The model under review builds one solid part; all positions refer to its coordinate system, in mm. Face numbers are marked on the shaded views. A direction names the side the tool comes from. Round coordinates to 2 decimals unless told otherwise and drop trailing zeros. Write each loop counter-clockwise with the first axis right and the second up, starting at its lowest first coordinate (ties: lowest second). Pieces come first, ordered by that corner, then holes. Notation, with made-up numbers: (24.5, 77) -> (80.5, 77) arc R15 ccw to (80.5, 95) -> close; hole circle Ø7 at (21.5, 84.25). An arc over 180 degrees is marked (long way). Answer in a Markdown table with one row per item. Add a question column.
```python
from build123d import *

# Parameters (mm, degrees)
F0_W     = 60.6719590724
F0_H     = 22.7290727198
F1_DEPTH = 44.45
F2_T     = -5.08
F4_DEPTH = 5.08
F6_DEPTH = 5.08
F7_R     = 2.6371182677
F8_DEPTH = 55.245


with BuildPart() as f1:
    # F0 (on Front) → F1 (new body)
    with BuildSketch(Plane.XZ):
        with Locations((-0.4582479596, -0.0916495919)):
            Rectangle(F0_W, F0_H)
    extrude(amount=F1_DEPTH)

    # F2
    f2_openings = [f1.faces().sort_by_distance(p)[0] for p in [
        (-0.458248, -22.225, 11.272887),
    ]]
    offset(amount=F2_T, openings=f2_openings)

    # F3 (on face) → F4 (join)
    with BuildSketch(Plane.YZ.offset(29.8777315766)):
        Polygon((-23.583047092, 26.9575025886), (-44.45, 11.272886768), (0, 11.272886768), align=None)
    extrude(amount=-F4_DEPTH)

    # F5 (on face) → F6 (join)
    with BuildSketch(Plane(origin=(-30.7942274958, 0, 0), x_dir=(0, -1, 0), z_dir=(-1, 0, 0))):
        Polygon((23.8014105707, 26.3420511037), (0, 11.272886768), (44.45, 11.272886768), align=None)
    extrude(amount=-F6_DEPTH)

    # F7 (on face) → F8 (join)
    with BuildSketch(Plane.YZ.offset(-25.7142274958)):
        with Locations((-23.0470523238, 16.2523370236)):
            Circle(F7_R)
    extrude(amount=F8_DEPTH)


solid = f1.part
```
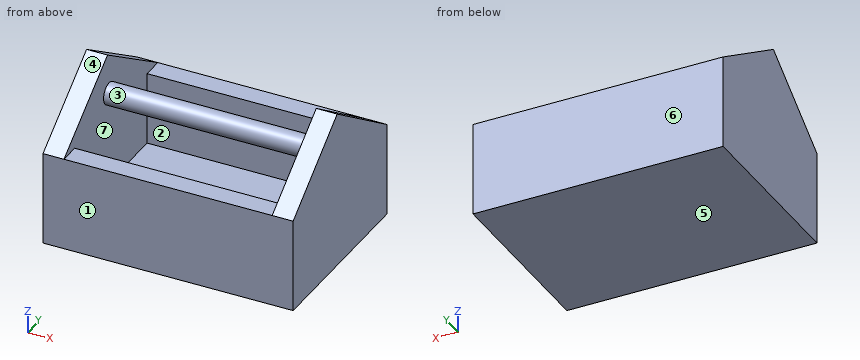
1. Mouldability with a two-part tool opening along Z and no side actions: class the marked faces 5, 6 and 7 as pulls with the +Z half, pulls with the -Z half, needs draft (parallel to the pull), parting line crosses it, or undercut.
2. Add section D-D on z = 12. Write out the cut boundary in (x, y).
3. Tool access review of the marked faces 1, 2, 3 and 4: name each direction out of +Z, -Z, +X, -X, +Y, -Y from which nothing blocks a thin tool from reaching the whole face with its end or side.
4. Add section B-B on y = -24.5. Write out the cut boundary in (x, z), plus the area to 3 significant figures.
5. Add section A-A on z = 4. Write out the cut boundary in (x, y).
6. Insertion check: pin 1 Ø4 at (x, y) = (-5, -41) entering from +Z; pin 2 Ø17 at (x, y) = (2.5, -26) entering from +Z. Each pin has a flat end and moves straight along its axis. Give the tip position at first contact, or say it passes through.
7. Add section C-C on x = -2. Write out the cut boundary in (y, z), plus the area to 3 significant figures.
8. For L1, parallel to X at y = -35.5, z = -3.5; L2, parallel to Y at x = -7, z = 9.5; L3, parallel to Z at x = 7.5, y = -37, list the stretches that pass through material, from the lowest coordinate up.
Filled in:
| question | item | result |
|---|---|---|
| 1 | face 5 | pulls with the -Z half |
| 1 | face 6 | needs draft |
| 1 | face 7 | undercut |
| 2 | outline | (-30.79, -43.45) -> (-25.71, -43.45) -> (-25.71, -1.15) -> (-30.79, -1.15) -> close; (24.8, -43.48) -> (29.88, -43.48) -> (29.88, -1.09) -> (24.8, -1.09) -> close |
| 3 | face 1 | +Z, -Z, +X, -X, -Y |
| 3 | face 2 | +Z |
| 3 | face 3 | none |
| 3 | face 4 | +Z, -X, -Y |
| 4 | outline | (-30.79, -11.46) -> (29.88, -11.46) -> (29.88, 26.27) -> (24.8, 26.27) -> (24.8, 18.45) -> (-25.71, 18.45) -> (-25.71, 25.83) -> (-30.79, 25.83) -> close; hole (-25.71, -6.38) -> (24.8, -6.38) -> (24.8, 14.05) -> (-25.71, 14.05) -> close |
| 4 | area | 860 mm² |
| 5 | outline | (-30.79, -44.45) -> (29.88, -44.45) -> (29.88, 0) -> (-30.79, 0) -> close; hole (-25.71, -39.37) -> (24.8, -39.37) -> (24.8, -5.08) -> (-25.71, -5.08) -> close |
| 6 | pin 1 | z = 11.27 |
| 6 | pin 2 | z = 18.89 |
| 7 | outline | (-44.45, -11.46) -> (0, -11.46) -> (0, 11.27) -> (-5.08, 11.27) -> (-5.08, -6.38) -> (-39.37, -6.38) -> (-39.37, 11.27) -> (-44.45, 11.27) -> close; circle Ø5.27 at (-23.05, 16.25) |
| 7 | area | 427 mm² |
| 8 | L1 | -30.79 to -25.71, 24.8 to 29.88 |
| 8 | L2 | -44.45 to -39.37, -5.08 to 0 |
| 8 | L3 | -11.46 to -6.38 |
